```python
from build123d import *

# Parameters (mm, degrees)
SKETCH1_W           = 12
SKETCH1_H           = 6
BOSS_EXTRUDE1_DEPTH = 13
SKETCH2_W           = 1
SKETCH2_H           = 2
BOSS_EXTRUDE2_DEPTH = 1.5
SKETCH3_W           = 11
SKETCH3_H           = 4
CUT_EXTRUDE1_DEPTH  = 5
SKETCH4_W           = 11
SKETCH4_H           = 1
CUT_EXTRUDE2_DEPTH  = 2
SKETCH5_R           = 0.25
BOSS_EXTRUDE3_DEPTH = 3


with BuildPart() as part:
    # Sketch1 → Boss-Extrude1 (new body)
    with BuildSketch(Plane(origin=(0, 0, 0), x_dir=(1, 0, 0), z_dir=(0, 1, 0))):
        Rectangle(SKETCH1_W, SKETCH1_H)
    extrude(amount=BOSS_EXTRUDE1_DEPTH)

    # Sketch2 → Boss-Extrude2 (add)
    with BuildSketch(Plane(origin=(6, 0, 0), x_dir=(0, 0, -1), z_dir=(1, 0, 0))):
        with Locations((2.5, 1)):
            Rectangle(SKETCH2_W, SKETCH2_H)
        with Locations((-2.5, 1)):
            Rectangle(SKETCH2_W, SKETCH2_H)
    boss_extrude2 = extrude(amount=BOSS_EXTRUDE2_DEPTH)

    # Mirror1: Boss-Extrude2 across plane
    add(boss_extrude2.mirror(Plane(origin=(0, 0, 0), x_dir=(0, 0, 1), z_dir=(1, 0, 0))))

    # Sketch3 → Cut-Extrude1 (cut)
    with BuildSketch(Plane(origin=(0, 13, 0), x_dir=(1, 0, 0), z_dir=(0, 1, 0))):
        Rectangle(SKETCH3_W, SKETCH3_H)
    extrude(amount=-CUT_EXTRUDE1_DEPTH, mode=Mode.SUBTRACT)

    # Sketch4 → Cut-Extrude2 (cut)
    with BuildSketch(Plane(origin=(0, 13, 0), x_dir=(1, 0, 0), z_dir=(0, 1, 0))):
        with Locations((0, 2.5)):
            Rectangle(SKETCH4_W, SKETCH4_H)
        with Locations((0, -2.5)):
            Rectangle(SKETCH4_W, SKETCH4_H)
    extrude(amount=-CUT_EXTRUDE2_DEPTH, mode=Mode.SUBTRACT)

    # Sketch5 → Boss-Extrude3 (add)
    with BuildSketch(Plane(origin=(0, 8, 0), x_dir=(1, 0, 0), z_dir=(0, 1, 0))):
        with Locations(Location((0, 1, 0), (0, 0, 270))):
            Circle(SKETCH5_R)
        with Locations(Location((2, 1, 0), (0, 0, 270))):
            Circle(SKETCH5_R)
        with Locations(Location((4, 1, 0), (0, 0, 270))):
            Circle(SKETCH5_R)
        with Locations(Location((-4, 1, 0), (0, 0, 90))):
            Circle(SKETCH5_R)
        with Locations(Location((-2, 1, 0), (0, 0, 90))):
            Circle(SKETCH5_R)
        with Locations(Location((4, -1, 0), (0, 0, 90))):
            Circle(SKETCH5_R)
        with Locations(Location((2, -1, 0), (0, 0, 90))):
            Circle(SKETCH5_R)
        with Locations(Location((0, -1, 0), (0, 0, 90))):
            Circle(SKETCH5_R)
        with Locations(Location((-2, -1, 0), (0, 0, 270))):
            Circle(SKETCH5_R)
        with Locations(Location((-4, -1, 0), (0, 0, 270))):
            Circle(SKETCH5_R)
    extrude(amount=BOSS_EXTRUDE3_DEPTH)


solid = part.part
```
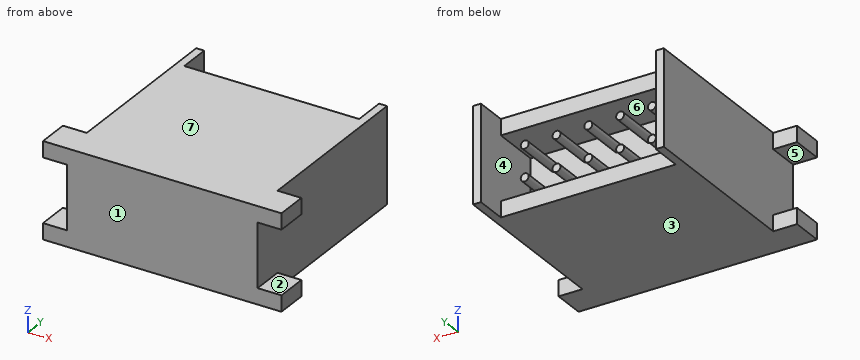
CAD build for the part. Positions are in the model's coordinates, mm. Face numbers are marked on the shaded views. A direction names the side the tool comes from. Coordinates: 2 decimals unless noted, no trailing zeros. Order: outer loops, then holes, each group sorted by start corner. A loop starts at its lowest first (then second) coordinate and runs counter-clockwise, first axis right, second up. Notation, with made-up numbers: (28.5, 79) - (33.5, 79) arc R29 ccw to (33.5, 116) - close; hole circle Ø7 at (46.25, 74). An arc over 180 degrees is marked (long way). Use a Markdown table: item, result. Add a question column.
(1) Which spindle directions (+Z, -Z, +X, -X, +Y, -Y) get a long thin tool onto all of the face, cutting with end or side? Do the marked faces 1, 2, 3, 4 and 5. Say none if no direction does.
(2) Saw through at A-A (z = 1.65). Give the cut face in (x, y), then the cut area to 3 significant figures.
(3) Saw through at B-B (x = 4). Give the cut face in (y, z), then the cut area to 3 significant figures.
(4) Flat gauge pins, fed straight in: pin 1 (2 mm diameter, centred on y = 7.5, z = 2, fed in from -X); pin 2 (0.6 mm diameter, centred on x = 2, z = 1, fed in from +Y); pin 3 (0.8 mm diameter, centred on x = 6.5, z = -2.5, fed in from +Y). Where does each tip first touch, or does it go through?
(5) Pull direction X, two halves, no side cores. Call the marked faces 6 and 7: +X half, -X half, draft (parallel to the pull), parting line (faces both ways), or undercut.
(6) Drill centre lines: line 1 along Y through (x, z) = (0.75, 2.35); line 2 along Y through (x, z) = (1, -1.8); line 3 along X through (y, z) = (10.5, 1.3). Where is each one in solid material? Low to high. Write a range as [from, to].
(7) Saw through at D-D (z = -2.3). Give the cut face in (x, y).
(8) Saw through at C-C (y = 4.75). Give the cut face in (x, z).
Solved:
| question | item | result |
|---|---|---|
| 1 | face 1 | +Z, -Z, +X, -X, -Y |
| 1 | face 2 | +X, +Y, -Y |
| 1 | face 3 | -Z, +X, -X, +Y, -Y |
| 1 | face 4 | +Y |
| 1 | face 5 | -X, +Y, -Y |
| 2 | outline | (-6, 0) - (6, 0) - (6, 13) - (5.5, 13) - (5.5, 8) - (-5.5, 8) - (-5.5, 13) - (-6, 13) - close |
| 2 | area | 101 mm² |
| 3 | outline | (0, -3) - (11, -3) - (11, -2) - (8, -2) - (8, -1.25) - (11, -1.25) - (11, -0.75) - (8, -0.75) - (8, 0.75) - (11, 0.75) - (11, 1.25) - (8, 1.25) - (8, 2) - (11, 2) - (11, 3) - (0, 3) - close |
| 3 | area | 57.0 mm² |
| 4 | pin 1 | stops at x = -6 |
| 4 | pin 2 | stops at y = 11 |
| 4 | pin 3 | stops at y = 2 |
| 5 | face 6 | undercut |
| 5 | face 7 | draft |
| 6 | line 1 | y = [0, 11] |
| 6 | line 2 | y = [0, 8] |
| 6 | line 3 | x = [-6, -5.5], [5.5, 6] |
| 7 | outline | (-7.5, 0) - (7.5, 0) - (7.5, 2) - (6, 2) - (6, 13) - (5.5, 13) - (5.5, 11) - (-5.5, 11) - (-5.5, 13) - (-6, 13) - (-6, 2) - (-7.5, 2) - close |
| 8 | outline | (-6, -3) - (6, -3) - (6, 3) - (-6, 3) - close |
